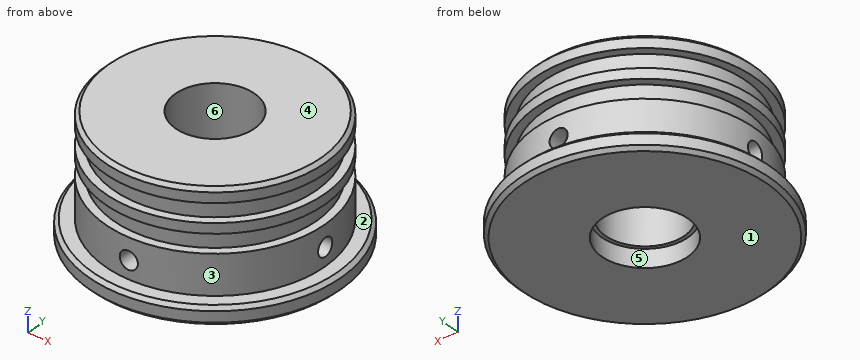
```python
from build123d import *

# Parameters (mm, degrees)
SKETCH_1_R               = 17.5
SKETCH_1_R_2             = 5.5
EXTRUDE_1_DEPTH          = 2.5
EXTRUDE_START            = 14
SKETCH_1_3_R             = 15.25
SKETCH_1_3_R_2           = 5.5
EXTRUDE_2_DEPTH          = 14
CUT_EXTRUDE_START        = 8.1
SKETCH_1_4_R             = 15.25
SKETCH_1_4_R_2           = 14.1
CUT_EXTRUDE_1_DEPTH      = 2.6
CUT_EXTRUDE_START_2      = 12.1
SKETCH_1_5_R             = 15.25
SKETCH_1_5_R_2           = 14.1
CUT_EXTRUDE_2_DEPTH      = 2.6
CHAMFER_1_SIZE           = 0.5
SKETCH_2_R               = 6
CUT_EXTRUDE_3_DEPTH      = 2.5
CUT_EXTRUDE_START_3      = 10
SKETCH_3_R               = 1.25
CUT_EXTRUDE_4_DEPTH      = 10
PATTERN_CIRCULAR_1_COUNT = 4


with BuildPart() as part:
    # Sketch 1 → Extrude 1 (new body)
    with BuildSketch(Plane.XY):
        Circle(SKETCH_1_R)
        Circle(SKETCH_1_R_2, mode=Mode.SUBTRACT)
    extrude(amount=-EXTRUDE_1_DEPTH)

    # Sketch 1_3 → Extrude 2 (add)
    with BuildSketch(Plane.XY.offset(EXTRUDE_START)):
        Circle(SKETCH_1_3_R)
        Circle(SKETCH_1_3_R_2, mode=Mode.SUBTRACT)
    extrude(amount=-EXTRUDE_2_DEPTH)

    # Sketch 1_4 → Cut-Extrude 1 (cut)
    with BuildSketch(Plane.XY.offset(CUT_EXTRUDE_START)):
        Circle(SKETCH_1_4_R)
        Circle(SKETCH_1_4_R_2, mode=Mode.SUBTRACT)
    extrude(amount=-CUT_EXTRUDE_1_DEPTH, mode=Mode.SUBTRACT)

    # Sketch 1_5 → Cut-Extrude 2 (cut)
    with BuildSketch(Plane.XY.offset(CUT_EXTRUDE_START_2)):
        Circle(SKETCH_1_5_R)
        Circle(SKETCH_1_5_R_2, mode=Mode.SUBTRACT)
    extrude(amount=-CUT_EXTRUDE_2_DEPTH, mode=Mode.SUBTRACT)

    # Chamfer 1
    chamfer_1_edges = [part.edges().sort_by_distance(p)[0] for p in [
        (-15.25, 0, 14),
        (-17.5, 0, 0),
        (-17.5, 0, -2.5),
    ]]
    chamfer(chamfer_1_edges, length=CHAMFER_1_SIZE)

    # Sketch 2 → Cut-Extrude 3 (cut)
    with BuildSketch(Plane(origin=(0, 0, -2.5), x_dir=(-1, 0, 0), z_dir=(0, 0, -1))):
        Circle(SKETCH_2_R)
    extrude(amount=-CUT_EXTRUDE_3_DEPTH, mode=Mode.SUBTRACT)

    # Sketch 3 → Cut-Extrude 4 (cut)
    with BuildSketch(Plane(origin=(0, 0, 0), x_dir=(1, 0, 0), z_dir=(0, 1, 0)).offset(CUT_EXTRUDE_START_3)):
        with Locations(Location((0, -2.5, 0), (0, 0, 90))):
            Circle(SKETCH_3_R)
    cut_extrude_4 = extrude(amount=CUT_EXTRUDE_4_DEPTH, mode=Mode.SUBTRACT)

    # Pattern Circular 1: Cut-Extrude 4 ×4 about axis
    pattern_circular_1_axis = Axis((0, 0, 0), (0, 0, 1))
    for i in range(1, PATTERN_CIRCULAR_1_COUNT):
        add(cut_extrude_4.rotate(pattern_circular_1_axis, i * 360 / PATTERN_CIRCULAR_1_COUNT), mode=Mode.SUBTRACT)


solid = part.part
```
Work out the finished part from the listing and answer in its coordinate system (mm). Face numbers are marked on the shaded views. A direction names the side the tool comes from. Coordinates: 2 decimals unless noted, no trailing zeros. Write each loop counter-clockwise with the first axis right and the second up, starting at its lowest first coordinate (ties: lowest second). Pieces come first, ordered by that corner, then holes.
Q1. Which of the six approach directions +Z, -Z, +X, -X, +Y, -Y give full straight-line access (tool end or side, diameter ignored) to the marked faces 1 and 2?
Q2. A cutting plane is placed at A-A, the plane z = 2.5. Give the vertices of the cut face in (x, y).
Q3. Find the intervals of material crossed by line 1 (Z direction, x = -8, y = -12); line 2 (Y direction, x = 0, z = 7); line 3 (Y direction, x = 0, z = -0.9), in increasing order.
Q4. Each of these flat-tipped pins is pushed along its axis until it touches: pin 1 Ø1.5 at (y, z) = (-8.5, 11) entering from -X; pin 2 Ø0.8 at (y, z) = (-0.5, 2.5) entering from -X; pin 3 Ø1 at (y, z) = (5.5, 7.5) entering from -X; pin 4 Ø1 at (x, y) = (3, 1) entering from -Z. Where does it stop, or does it pass through?
Q5. Determine the mould class of the marked faces 3, 4, 5 and 6 for opening direction Y: released by +Y, released by -Y, zero draft, split by the parting line, or undercut.
Findings below:
1. face 1: -Z, +X, -X, +Y, -Y
1. face 2: +Z
2. outline: (-15.2, -1.25) arc R15.25 ccw to (-1.25, -15.2) - (-1.25, -10) - (1.25, -10) - (1.25, -15.2) arc R15.25 ccw to (15.2, -1.25) - (10, -1.25) - (10, 1.25) - (15.2, 1.25) arc R15.25 ccw to (1.25, 15.2) - (1.25, 10) - (-1.25, 10) - (-1.25, 15.2) arc R15.25 ccw to (-15.2, 1.25) - (-10, 1.25) - (-10, -1.25) - close; hole circle Ø11 at (0, 0)
3. line 1: z = -2.5 to 5.5, 8.1 to 9.5, 12.1 to 14
3. line 2: y = -14.1 to -5.5, 5.5 to 14.1
3. line 3: y = -17.5 to -6, 6 to 17.5
4. pin 1: stops at x = -11.78
4. pin 2: stops at x = -10
4. pin 3: stops at x = -13.18
4. pin 4: passes through
5. face 3: split by the parting line
5. face 4: zero draft
5. face 5: undercut
5. face 6: undercut
